The listing builds one solid part. Answer for the finished solid, in the listing's coordinates (mm). Round coordinates to 2 decimals unless told otherwise and drop trailing zeros. Write each loop counter-clockwise with the first axis right and the second up, starting at its lowest first coordinate (ties: lowest second). Pieces come first, ordered by that corner, then holes. Notation, with made-up numbers: (-11.5, 37.25) - (44.5, 37.25) arc R33 cw to (44.5, 68.25) - close; hole circle Ø7 at (16, 30). An arc over 180 degrees is marked (long way). Return JSON: item names as keys, results as strings. Group by question number.
(1) Section C-C, the plane z = -12.5 is taken. Write down the section's boundary in (x, y).
(2) Section B-B, the plane y = -7.5 is taken. Write down the section's boundary in (x, z), then the cut area to 3 significant figures.
(3) Each of these flat-tipped pins is pushed along its axis until it touches: pin 1 (0.8 mm diameter, centred on x = 1.5, z = 29, fed in from -Y); pin 2 (3 mm diameter, centred on y = 3, z = 19.5, fed in from -X); pin 3 (0.8 mm diameter, centred on y = -0.5, z = 29, fed in from -X); pin 4 (1.5 mm diameter, centred on y = 0.5, z = -10.5, fed in from +X). Where does it stop, or does it pass through?
(4) Find the intervals of material crossed by line 1 along Y through (x, z) = (1.7, -16.5); line 2 along Z through (x, y) = (1.7, -1); line 3 along Z through (x, y) = (1.5, 0.25), in increasing order. Write a range as [from, to].
(5) Section A-A, the plane z = -6.5 is taken. Write down the section's boundary in (x, y).
(6) Section D-D, the plane y = -1.5 is taken. Write down the section's boundary in (x, z).
Autodesk Inventor part; units mm, degrees
ref_plane "YZ Plane" through (0, 0, 0) normal (1, 0, 0) x (0, 1, 0)
ref_plane "XZ Plane" through (0, 0, 0) normal (0, 1, 0) x (-1, 0, 0)
ref_plane "XY Plane" through (0, 0, 0) normal (0, 0, 1) x (1, 0, 0)
sketch "스케치1" plane through (0, 0, 0) normal (1, 0, 0) x (0, 1, 0)
  line L0 (10.5, 28) -> (-10.5, 28)
  line L1 (-10.5, 28) -> (-10.5, -28)
  line L2 (-10.5, -28) -> (10.5, -28)
  line L3 (10.5, -28) -> (10.5, 28)
  line L4 (10.5, 28) -> (-10.5, -28) construction
  line L5 (-10.5, 28) -> (10.5, -28) construction
  point P0 (0, 0)
  dimension "d0" = 21
  dimension "d1" = 56
extrude "돌출1" add sketch "스케치1" along normal blind 2.7
sketch "스케치2" plane through (0, -10.5, 28) normal (0, 0, 1) x (1, 0, 0)
  line L0 (0.31, 12) -> (2.01, 12)
  line L1 (2.01, 12) -> (2.01, 7)
  line L2 (2.01, 7) -> (0.31, 7)
  line L3 (0.31, 7) -> (0.31, 12)
  line L4 (0.31, 12) -> (2.01, 7) construction
  line L5 (2.01, 12) -> (0.31, 7) construction
  line L6 (-0.39, -0.5) -> (-0.39, 15)
  line L7 (-0.39, -0.5) -> (2.9, -0.5)
  line L8 (2.7, 0) -> (2.7, 21)
  line L9 (0, 0) -> (2.7, 0)
  point P0 (0, 10.5)
  point P1 (35, -7)
  point P2 (1.16, 9.5)
  dimension "d4" = 1.7
  dimension "d5" = 5
  dimension "d6" = 0.7
  dimension "d8" = 0.69
  dimension "d21" = 9.5
extrude "돌출2" add sketch "스케치2" along normal blind 1.95
chamfer "모따기1" distance 0.5 angle 45 8 edges at (0, -10.5, 0) (0, 0, 28) (0, 10.5, 0) (0, 0, -28) (2.01, -1, 29.95) (1.16, 1.5, 29.95) (0.31, -1, 29.95) (1.16, -3.5, 29.95)
sketch "스케치3" plane through (0, 0, 0) normal (0, 1, 0) x (-1, 0, 0)
  line L0 (-2.7, 28) -> (-2.7, -28)
  line L1 (-2.7, -7.4045) -> (-0.7, -3.9404)
  line L2 (-0.7, -3.9404) -> (-0.7, -19.4045)
  line L3 (-0.7, -19.4045) -> (-2.7, -19.4045)
  line L4 (-2.7, -19.4045) -> (-2.7, -7.4045)
  point P0 (0, 0)
  dimension "d18" = 12
  dimension "d19" = 30
  dimension "d20" = 2
extrude "돌출4" cut sketch "스케치3" along normal mid plane 5
properties part number "bt cover"
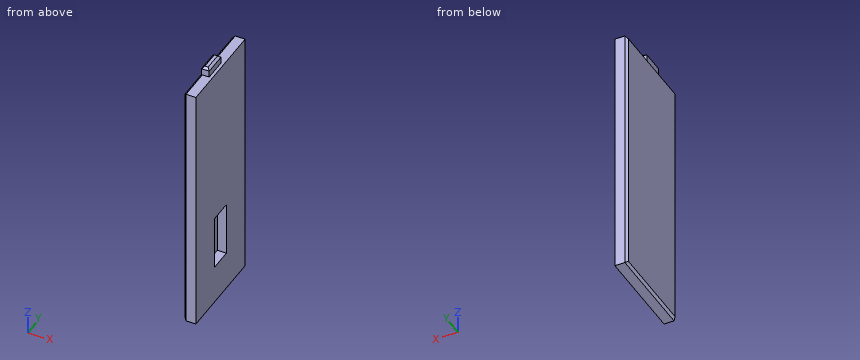
Working result:
{
 "1": {"outline": "(0, -10) - (0.5, -10.5) - (2.7, -10.5) - (2.7, -2.5) - (0.7, -2.5) - (0.7, 2.5) - (2.7, 2.5) - (2.7, 10.5) - (0.5, 10.5) - (0, 10) - close"},
 "2": {"outline": "(0, -27.5) - (0.5, -28) - (2.7, -28) - (2.7, 28) - (0.5, 28) - (0, 27.5) - close", "area": "151 mm^2"},
 "3": {"pin 1": "stops at y = -3.5", "pin 2": "stops at x = 0", "pin 3": "stops at x = 0.31", "pin 4": "stops at x = 0.7"},
 "4": {"line 1": "y = [-10.5, -2.5], [2.5, 10.5]", "line 2": "z = [-28, -19.4], [-5.67, 29.76]", "line 3": "z = [-28, -19.4], [-5.33, 29.95]"},
 "5": {"outline": "(0, -10) - (0.5, -10.5) - (2.7, -10.5) - (2.7, 10.5) - (0.5, 10.5) - (0, 10) - close; hole (0.7, -2.5) - (2.18, -2.5) - (2.18, 2.5) - (0.7, 2.5) - close"},
 "6": {"outline": "(0, -27.5) - (0.5, -28) - (2.7, -28) - (2.7, -19.4) - (0.7, -19.4) - (0.7, -3.94) - (2.7, -7.4) - (2.7, 28) - (2.01, 28) - (2.01, 29.45) - (1.51, 29.95) - (0.81, 29.95) - (0.31, 29.45) - (0.31, 27.81) - (0, 27.5) - close"}
}
